Part print with two shaded views. Sizes in mm from the minimum x, y, z corner. A direction names the side the tool comes from. Round coordinates to 2 decimals unless told otherwise and drop trailing zeros. Loops run counter-clockwise (first coordinate to the right, second up) from the corner with the lowest first, then second, coordinate; pieces in that order, holes last. Notation, with made-up numbers: M -37.5,-34.75 L 3.5,-34.75 A4 cw 3.5,-30.75 Z; hole C 19.5,19 d9. An arc over 180 degrees is marked long. Put each result on its own line as item: value. Start each with the question number.
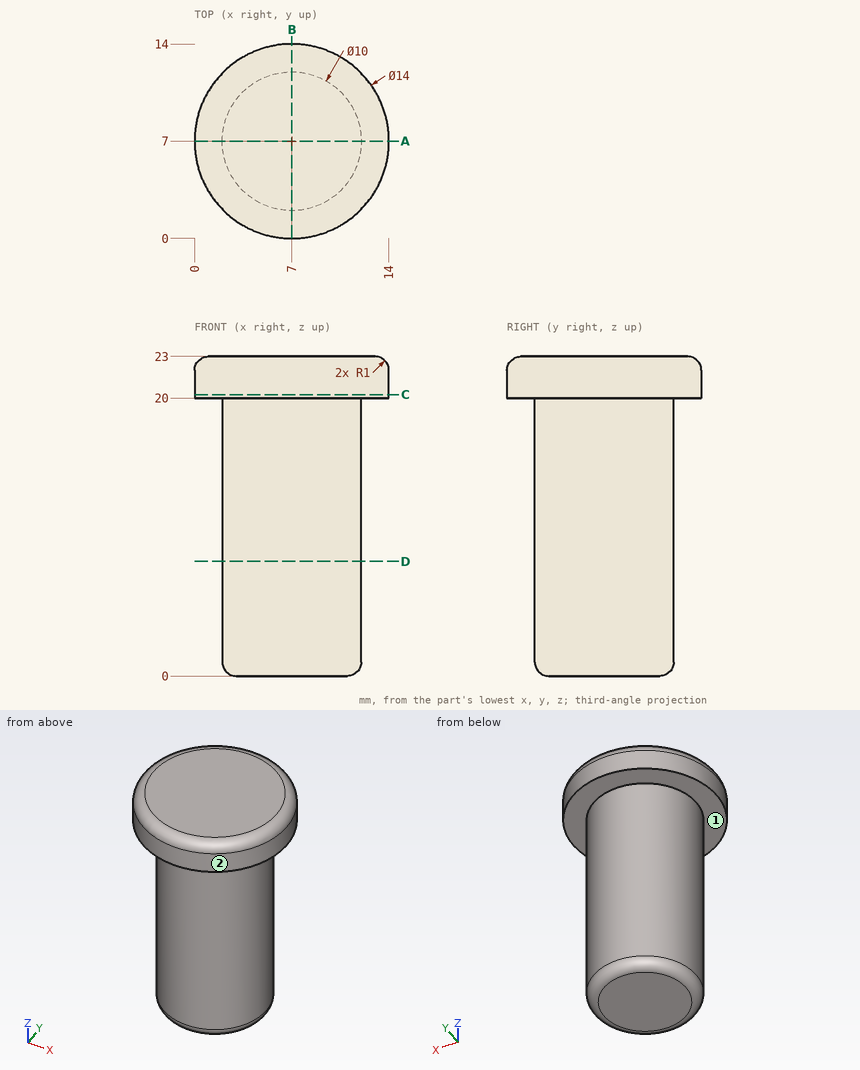
(1) Tool access for the marked faces 1 and 2: list every direction of +Z, -Z, +X, -X, +Y, -Y with a clear straight run to the whole face (end or side of a thin tool).
(2) Cut at D-D on z = 8.25. List the corners of the cut face in (x, y), and give its area (3 significant figures).
(3) Flat gauge pins, fed straight in: pin 1 Ø1.5 at (y, z) = (4, 5) entering from +X; pin 2 Ø3 at (x, z) = (7, 14) entering from +Y; pin 3 Ø1.5 at (x, z) = (9.5, 10) entering from +Y. Where does each tip first touch, or does it go through?
(4) Drill centre lines: line 1 along Z through (x, y) = (7.5, 13); line 2 along Z through (x, y) = (7.75, 11); line 3 along X through (y, z) = (3.25, 9.75). Where is each one in solid material? Low to high.
(5) Cut at A-A on y = 7. List the corners of the cut face in (x, z).
(6) Cut at C-C on z = 20.25. List the corners of the cut face in (x, y).
Taken from the geometry:
1. face 1: -Z
1. face 2: +Z, -Z
2. outline: C 7,7 d10
2. area: 78.5 mm2
3. pin 1: x = 11.47
3. pin 2: y = 12
3. pin 3: y = 11.68
4. line 1: 20 to 23
4. line 2: 0 to 23
4. line 3: 3.69 to 10.31
5. outline: M 0,20 L 2,20 L 2,1 A1 ccw 3,0 L 11,0 A1 ccw 12,1 L 12,20 L 14,20 L 14,22 A1 ccw 13,23 L 1,23 A1 ccw 0,22 Z
6. outline: C 7,7 d14
